```python
from build123d import *

# Parameters (mm, degrees)
SKETCH1_W               = 170
SKETCH1_H               = 150
BOSS_EXTRUDE1_DEPTH     = 3
SKETCH2_W               = 170
SKETCH2_H               = 3
BOSS_EXTRUDE3_DEPTH     = 10
SKETCH3_W               = 35
SKETCH3_H               = 3
BOSS_EXTRUDE4_DEPTH     = 30
FILLET1_R               = 17.5
FILLET1_OF_MIRROR2_R    = 17.5
MIRROR3_START           = -75
MIRROR3_DEPTH           = 3
SKETCH7_W               = 70
SKETCH7_H               = 90
CUT_EXTRUDE1_DEPTH      = 3
SKETCH12_R              = 6
CUT_EXTRUDE2_DEPTH      = 175.453432182
BOSS_EXTRUDE5_DEPTH     = 3
FILLET2_R               = 2
FILLET3_R               = 2
FILLET2_OF_MIRROR5_R    = 2
FILLET3_OF_MIRROR5_R    = 2
SKETCH13_W              = 186.373128994
SKETCH13_H              = 150
BOSS_EXTRUDE6_DEPTH     = 3
SKETCH14_W              = 15
SKETCH14_H              = 15
SKETCH14_W_2            = 13
SKETCH14_H_2            = 13
BOSS_EXTRUDE8_DEPTH     = 210
SKETCH16_W              = 45.036207967
SKETCH16_H              = 34.729984481
BOSS_EXTRUDE9_DEPTH     = 3
CUT_EXTRUDE3_DEPTH      = 10
CUT_EXTRUDE3_DEPTH_BACK = 150
SKETCH17_W              = 3
SKETCH17_H              = 185.851643629
SKETCH18_R              = 35
CUT_EXTRUDE4_DEPTH      = 44
CUT_EXTRUDE6_DEPTH      = 2
CUT_EXTRUDE6_DEPTH_BACK = 17
SKETCH19_W              = 29.178069821
SKETCH19_H              = 150


# Read off the part's stored shape, not the designer's step: Mirror3
with BuildPart() as part:
    # Sketch1 → Boss-Extrude1 (new body)
    with BuildSketch(Plane.XY):
        Rectangle(SKETCH1_W, SKETCH1_H)
    extrude(amount=BOSS_EXTRUDE1_DEPTH)

    # Sketch2 → Boss-Extrude3 (add)
    with BuildSketch(Plane(origin=(0, 0, 0), x_dir=(-1, 0, 0), z_dir=(0, 0, -1))):
        with Locations((0, 73.5)):
            Rectangle(SKETCH2_W, SKETCH2_H)
        with Locations((0, -73.5)):
            Rectangle(SKETCH2_W, SKETCH2_H)
    extrude(amount=BOSS_EXTRUDE3_DEPTH)

    # Sketch3 → Boss-Extrude4 (add)
    with BuildSketch(Plane(origin=(0, 0, -10), x_dir=(-1, 0, 0), z_dir=(0, 0, -1))):
        with Locations((57.5, 73.5)):
            Rectangle(SKETCH3_W, SKETCH3_H)
    boss_extrude4 = extrude(amount=BOSS_EXTRUDE4_DEPTH)

    # Fillet1
    fillet1_edges = [part.edges().sort_by_distance(p)[0] for p in [
        (-40, 73.5, -40),
        (-75, 73.5, -40),
    ]]
    fillet(fillet1_edges, radius=FILLET1_R - 0.0001)  # a hair under: the kernel refuses the full size

    # Mirror2: Boss-Extrude4 across plane
    add(boss_extrude4.mirror(Plane(origin=(0, 0, 0), x_dir=(0, 0, 1), z_dir=(1, 0, 0))))

    # Fillet1 of Mirror2
    fillet1_of_mirror2_edges = [part.edges().sort_by_distance(p)[0] for p in [
        (40, 73.5, -40),
        (75, 73.5, -40),
    ]]
    fillet(fillet1_of_mirror2_edges, radius=FILLET1_OF_MIRROR2_R - 0.0001)  # a hair under: the kernel refuses the full size

    # Mirror3 outline → Mirror3 (add)
    with BuildSketch(Plane(origin=(0, 0, 0), x_dir=(1, 0, 0), z_dir=(0, 1, 0)).offset(MIRROR3_START)):
        with BuildLine():
            ThreePointArc((-57.5, 40), (-69.874368671, 34.874368671), (-75, 22.5))
            Line((-75, 22.5), (-75, 10))
            Line((-75, 10), (-40, 10))
            Line((-40, 10), (-40, 22.5))
            ThreePointArc((-40, 22.5), (-45.125631329, 34.874368671), (-57.5, 40))
        make_face()
        with BuildLine():
            Line((40, 22.5), (40, 10))
            Line((40, 10), (75, 10))
            Line((75, 10), (75, 22.5))
            ThreePointArc((75, 22.5), (69.874368671, 34.874368671), (57.5, 40))
            ThreePointArc((57.5, 40), (45.125631329, 34.874368671), (40, 22.5))
        make_face()
    extrude(amount=MIRROR3_DEPTH)

    # Sketch7 → Cut-Extrude1 (cut)
    with BuildSketch(Plane.XY.offset(3)):
        with Locations((-50, 0)):
            Rectangle(SKETCH7_W, SKETCH7_H)
        with Locations((50, 0)):
            Rectangle(SKETCH7_W, SKETCH7_H)
    extrude(amount=-CUT_EXTRUDE1_DEPTH, mode=Mode.SUBTRACT)

    # Sketch12 → Cut-Extrude2 (cut, symmetric)
    with BuildSketch(Plane.XZ.offset(-72)):
        with Locations((-57.5, -22.5)):
            Circle(SKETCH12_R)
    cut_extrude2 = extrude(amount=CUT_EXTRUDE2_DEPTH, both=True, mode=Mode.SUBTRACT)

    # Mirror4: Cut-Extrude2 across plane
    add(cut_extrude2.mirror(Plane(origin=(0, 0, 0), x_dir=(0, 0, 1), z_dir=(1, 0, 0))), mode=Mode.SUBTRACT)

    # Sketch10 → Boss-Extrude5 (add)
    with BuildSketch(Plane(origin=(0, 75, 0), x_dir=(1, 0, 0), z_dir=(0, 1, 0))):
        Polygon((15, -3), (-85, -3), (-85, -33), (115, -33), align=None)
    boss_extrude5 = extrude(amount=-BOSS_EXTRUDE5_DEPTH)

    # Fillet2
    fillet2_edges = [part.edges().sort_by_distance(p)[0] for p in [
        (115, 73.5, 33),
    ]]
    fillet(fillet2_edges, radius=FILLET2_R)

    # Fillet3
    fillet3_edges = [part.edges().sort_by_distance(p)[0] for p in [
        (15, 73.5, 3),
    ]]
    fillet(fillet3_edges, radius=FILLET3_R)

    # Mirror5: Boss-Extrude5 across plane
    add(boss_extrude5.mirror(Plane.ZX))

    # Fillet2 of Mirror5
    fillet2_of_mirror5_edges = [part.edges().sort_by_distance(p)[0] for p in [
        (115, -73.5, 33),
    ]]
    fillet(fillet2_of_mirror5_edges, radius=FILLET2_OF_MIRROR5_R)

    # Fillet3 of Mirror5
    fillet3_of_mirror5_edges = [part.edges().sort_by_distance(p)[0] for p in [
        (15, -73.5, 3),
    ]]
    fillet(fillet3_of_mirror5_edges, radius=FILLET3_OF_MIRROR5_R)

    # Sketch13 → Boss-Extrude6 (add)
    with BuildSketch(Plane.XY.offset(33)):
        with Locations((8.186564497, 0)):
            Rectangle(SKETCH13_W, SKETCH13_H)
    extrude(amount=BOSS_EXTRUDE6_DEPTH)

    # Sketch14 → Boss-Extrude8 (add)
    # profile 1 of 2: a face of its own
    with BuildSketch(Plane.XY.offset(36)):
        with Locations((28.873128994, -47.5)):
            Rectangle(SKETCH14_W, SKETCH14_H)
        with Locations((28.873128994, -47.5)):
            Rectangle(SKETCH14_W_2, SKETCH14_H_2, mode=Mode.SUBTRACT)
    # profile 2 of 2: a face of its own
    with BuildSketch(Plane.XY.offset(36)):
        Polygon((66.373128994, -55), (81.373128994, -55), (81.373128994, -40), (78.373128994, -40), (78.373128994, -52), (66.373128994, -52), align=None)
    boss_extrude8 = extrude(amount=BOSS_EXTRUDE8_DEPTH)

    # Mirror7: Boss-Extrude8 across plane
    add(boss_extrude8.mirror(Plane.ZX))

    # Sketch16 → Boss-Extrude9 (add)
    with BuildSketch(Plane.XZ.offset(55)):
        with Locations((58.855025011, 228.63500776)):
            Rectangle(SKETCH16_W, SKETCH16_H)
    boss_extrude9 = extrude(amount=BOSS_EXTRUDE9_DEPTH)

    # Mirror8: Boss-Extrude9 across plane
    add(boss_extrude9.mirror(Plane.ZX))

    # Sketch17 → Cut-Extrude3 (cut, two sides: drawn at the far end of the back side and taken through both)
    with BuildSketch(Plane(origin=(0, 55, 0), x_dir=(1, 0, 0), z_dir=(0, 1, 0)).offset(-CUT_EXTRUDE3_DEPTH_BACK)):
        with Locations((76.873128994, -138.999103357)):
            Rectangle(SKETCH17_W, SKETCH17_H)
    extrude(amount=CUT_EXTRUDE3_DEPTH + CUT_EXTRUDE3_DEPTH_BACK, mode=Mode.SUBTRACT)

    # Sketch18 → Cut-Extrude4 (cut)
    with BuildSketch(Plane.XY.offset(36)):
        with Locations((101.373128994, 0)):
            Circle(SKETCH18_R)
    extrude(amount=-CUT_EXTRUDE4_DEPTH, mode=Mode.SUBTRACT)

    # Sketch19 → Cut-Extrude6 (cut, two sides: drawn at the far end of the back side and taken through both)
    with BuildSketch(Plane.XY.offset(36).offset(-CUT_EXTRUDE6_DEPTH_BACK)):
        with Locations((97.511085228, 0)):
            Rectangle(SKETCH19_W, SKETCH19_H)
    extrude(amount=CUT_EXTRUDE6_DEPTH + CUT_EXTRUDE6_DEPTH_BACK, mode=Mode.SUBTRACT)


solid = part.part
```
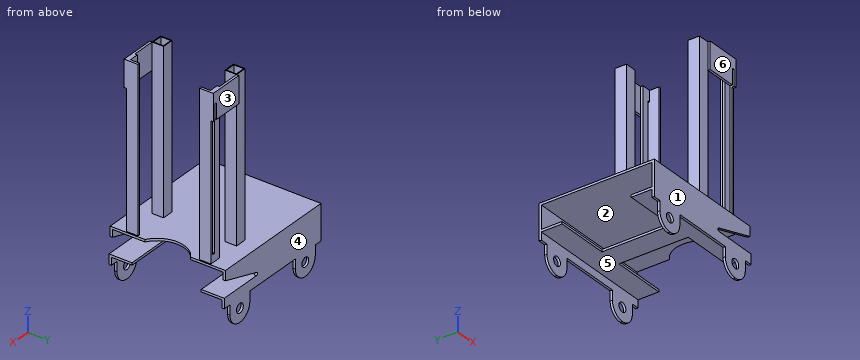
Part model, mm, in its own coordinate system. Face numbers are marked on the shaded views. A direction names the side the tool comes from. Coordinates: 2 decimals unless noted, no trailing zeros. Write each loop counter-clockwise with the first axis right and the second up, starting at its lowest first coordinate (ties: lowest second). Pieces come first, ordered by that corner, then holes.
Item 1: Slice it at B-B (y = -65). Write the cut outline in (x, z), and give its area (3 significant figures).
Item 2: Pin check, flat tips, straight feed: pin 1 (0.9 mm diameter, centred on y = -74, z = -14, fed in from +X); pin 2 (1.5 mm diameter, centred on x = 82, y = -74, fed in from -Z); pin 3 (1 mm diameter, centred on x = 53, y = -1, fed in from -Z); pin 4 (6.5 mm diameter, centred on y = 59.5, z = 27, fed in from +X). Stop position of each tip, or through.
Item 3: Which spindle directions (+Z, -Z, +X, -X, +Y, -Y) get a long thin tool onto all of the face, cutting with end or side? Do the marked faces 4, 5 and 6. Say none if no direction does.
Item 4: Mould opens along Y. For the marked faces 1, 2 and 3 say: released by +Y, released by -Y, zero draft, split by the parting line, or undercut.
Item 5: Slice it at A-A (z = 175). Count the separate pieces of the cut face and the enclosed holes in it, and give its area (3 significant figures).
Item 6: Probe line 1 (Y direction, x = 28.5, z = 219.5); line 2 (X direction, y = -43.5, z = 167); line 3 (Z direction, x = 38.5, y = 49). List the from-to ranges inside material, lowest first.
Item 7: Slice it at D-D (z = 30). Write the cut outline in (x, y), and give its area (3 significant figures).
Item 8: Slice it at C-C (x = 1.5). Write the cut outline in (y, z).
Results found:
1. outline: (-85, 0) - (85, 0) - (85, 3) - (-85, 3) - close; (-85, 33) - (82.92, 33) - (82.92, 36) - (-85, 36) - close
1. area: 1,010 mm2
2. pin 1: stops at x = 75
2. pin 2: stops at z = -10
2. pin 3: stops at z = 33
2. pin 4: passes through
3. face 4: +Z, -Z, +X, -X, +Y
3. face 5: -Z, +X, -X
3. face 6: +Z, +X, -X, -Y
4. face 1: released by -Y
4. face 2: undercut
4. face 3: released by +Y
5. separate pieces: 6
5. enclosed holes: 2
5. area: 256 mm2
6. line 1: y = -55 to -54, -41 to -40, 40 to 41, 54 to 55
6. line 2: x = 21.37 to 22.37, 35.37 to 36.37, 78.37 to 81.37
6. line 3: z = 0 to 3, 33 to 36
7. outline: (-85, -75) - (82.92, -75) - (82.92, -72) - (-85, -72) - close; (-85, 72) - (82.92, 72) - (82.92, 75) - (-85, 75) - close
7. area: 1,010 mm2
8. outline: (-75, -10) - (-72, -10) - (-72, 0) - (72, 0) - (72, -10) - (75, -10) - (75, 36) - (-75, 36) - close; hole (-72, 3) - (72, 3) - (72, 33) - (-72, 33) - close
